Autodesk Inventor part; units mm, degrees
ref_plane "YZ Plane" through (0, 0, 0) normal (1, 0, 0) x (0, 1, 0)
ref_plane "XZ Plane" through (0, 0, 0) normal (0, 1, 0) x (-1, 0, 0)
ref_plane "XY Plane" through (0, 0, 0) normal (0, 0, 1) x (1, 0, 0)
sketch "Sketch1" plane through (0, 0, 0) normal (0, 1, 0) x (-1, 0, 0)
  line L0 (-5.765, 13) -> (5.765, 13)
  line L1 (5.765, 13) -> (5.765, -13)
  line L2 (5.765, -13) -> (-5.765, -13)
  line L3 (-5.765, -13) -> (-5.765, 13)
  line L4 (-5.765, 13) -> (5.765, -13) construction
  line L5 (5.765, 13) -> (-5.765, -13) construction
  circle A0 centre (0, 9) radius 1.6
  circle A1 centre (0, -9) radius 1.6
  circle A2 centre (0, 9) radius 4
  circle A3 centre (0, -9) radius 4
  line L6 (5.765, 4) -> (3.8159, 10.1997)
  line L7 (3.8159, -10.1997) -> (5.765, -4)
  line L8 (-3.8159, -10.1997) -> (-5.765, -4)
  line L9 (-5.765, 4) -> (-3.8159, 10.1997)
  point P0 (0, 0)
  dimension "d0" = 26
  dimension "d1" = 11.53
  dimension "d2" = 18
  dimension "d3" = 9
  dimension "d4" = 3.2
  dimension "d5" = 8
  dimension "d6" = 4
  dimension "d7" = 4
extrude "Extrusion1" add sketch "Sketch1" along normal blind 2.3 contours A2 | L9 A2 L6 L1 L7 A3 L8 L3 | A3
sketch "Sketch2" plane through (0, 2.3, 0) normal (0, 1, 0) x (1, 0, 0)
  line L0 (5.765, -4) -> (5.765, 4)
  line L1 (5.765, 4) -> (3.8159, 10.1997)
  arc A0 (3.8159, 10.1997) -> (-3.8159, 10.1997) centre (0, 9) ccw
  line L2 (-3.8159, 10.1997) -> (-5.765, 4)
  line L3 (-5.765, 4) -> (-5.765, -4)
  line L4 (-5.765, -4) -> (-3.8159, -10.1997)
  arc A1 (-3.8159, -10.1997) -> (3.8159, -10.1997) centre (0, -9) ccw
  line L5 (3.8159, -10.1997) -> (5.765, -4)
  circle A2 centre (0, -9) radius 1.6
  circle A3 centre (0, 9) radius 1.6
  circle A4 centre (0, 0) radius 5
  dimension "d10" = 10
extrude "Extrusion2" add sketch "Sketch2" along normal blind 7.7 contours A4
sketch "Sketch3" plane through (0, 10, 0) normal (0, 1, 0) x (1, 0, 0)
  circle A0 centre (0, 0) radius 5
  line L0 (5.765, 6.5) -> (-5.765, 6.5)
  line L1 (-5.765, 6.5) -> (-5.765, -6.5)
  line L2 (-5.765, -6.5) -> (5.765, -6.5)
  line L3 (5.765, -6.5) -> (5.765, 6.5)
  line L4 (5.765, 6.5) -> (-5.765, -6.5) construction
  line L5 (-5.765, 6.5) -> (5.765, -6.5) construction
  circle A1 centre (0, 0) radius 6.5
  point P0 (-5.765, 4)
  point P1 (5.765, -3.0025)
  point P2 (5.765, 3.0025)
  point P3 (-5.765, 3.0025)
  point P4 (-5.765, -3.0025)
  dimension "d13" = 13
extrude "Extrusion3" add sketch "Sketch3" along normal blind 26.3 contours A0 | A1 L3 L1
sketch "Sketch4" plane through (0, 36.3, 0) normal (0, 1, 0) x (1, 0, 0)
  circle A0 centre (0, 0) radius 1
  dimension "d19" = 2
chamfer "Chamfer1" distance 3 angle 45 4 edges at (0, 36.3, -6.5) (0, 36.3, 6.5) (5.765, 36.3, 0) (-5.765, 36.3, 0)
extrude "Extrusion4" add sketch "Sketch4" along normal blind 3.7
properties part number "BLTouch" material "ABS Plastic"
CAD build for the part. Positions are in the model's coordinates, mm. A direction names the side the tool comes from. Coordinates: 2 decimals unless noted, no trailing zeros. Order: outer loops, then holes, each group sorted by start corner. A loop starts at its lowest first (then second) coordinate and runs counter-clockwise, first axis right, second up.
Item 1: Band-saw the part on D-D on y = 19.5. List the corners of the cut face in (x, z) (3 decimals).
Check sheet entries:
outline: (-5.765, -3.002) arc R6.5 ccw to (5.765, -3.002) - (5.765, 3.002) arc R6.5 ccw to (-5.765, 3.002) - close
Item 2: 3-axis set-ups, long thin cutter, end or side, ignore diameter. For faces 4 (the face through (0.1, 35.1, 4.7)), 5 (the face through (2, 10, 5)), 6 (the face through (-1, 36.3, -1)): which of +Z, -Z, +X, -X, +Y, -Y reach the whole face in a straight line?
Check sheet entries:
face 4: +Z, +Y
face 5: none
face 6: +Y
Item 3: Drill centre lines: L1, parallel to Z at x = 0, y = 1.55; L2, parallel to Y at x = 1.5, z = -2; L3, parallel to Y at x = -3.25, z = -5.5. Where is each one in solid material? Low to high.
Check sheet entries:
L1: z = -13 to -10.6, -7.4 to 7.4, 10.6 to 13
L2: y = 0 to 36.3
L3: y = 0 to 2.3, 10 to 33.41
Item 4: Pin check, flat tips, straight feed: pin 1 Ø1.5 at (x, y) = (3.5, 16) entering from +Z; pin 2 Ø5 at (x, y) = (-3, 14.5) entering from -Z; pin 3 Ø2 at (x, z) = (-3.5, -6.5) entering from +Y. Stop position of each tip, or through.
Check sheet entries:
pin 1: stops at z = 5.89
pin 2: stops at z = -6.48
pin 3: stops at y = 33.42
Item 5: Band-saw the part on A-A on x = 0. List the corners of the cut face in (y, z).
Check sheet entries:
outline: (0, -13) - (2.3, -13) - (2.3, -10.6) - (0, -10.6) - close; (0, -7.4) - (2.3, -7.4) - (2.3, -5) - (10, -5) - (10, -6.5) - (33.3, -6.5) - (36.3, -3.5) - (36.3, -1) - (40, -1) - (40, 1) - (36.3, 1) - (36.3, 3.5) - (33.3, 6.5) - (10, 6.5) - (10, 5) - (2.3, 5) - (2.3, 7.4) - (0, 7.4) - close; (0, 10.6) - (2.3, 10.6) - (2.3, 13) - (0, 13) - close
Item 6: Two-plate mould, pull along Y, no slides. Class faces 1 (the face through (4.286, 34.779, 0.042)), 2 (the face through (5.2, 2.3, 0.2)), 3 (the face through (0, 0, 0)): +Y half, -Y half, draft (parallel to the pull), parting line (faces both ways), or undercut.
Check sheet entries:
face 1: +Y half
face 2: undercut
face 3: -Y half
Item 7: Band-saw the part on B-B on z = -9. List the corners of the cut face in (x, y).
Check sheet entries:
outline: (-4.19, 0) - (-1.6, 0) - (-1.6, 2.3) - (-4.19, 2.3) - close; (1.6, 0) - (4.19, 0) - (4.19, 2.3) - (1.6, 2.3) - close
Item 8: Band-saw the part on C-C on z = 0. List the corners of the cut face in (x, y) (3 decimals).
Check sheet entries:
outline: (-5.765, 0) - (5.765, 0) - (5.765, 2.3) - (5, 2.3) - (5, 10) - (5.765, 10) - (5.765, 33.3) - (2.765, 36.3) - (1, 36.3) - (1, 40) - (-1, 40) - (-1, 36.3) - (-2.765, 36.3) - (-5.765, 33.3) - (-5.765, 10) - (-5, 10) - (-5, 2.3) - (-5.765, 2.3) - close
